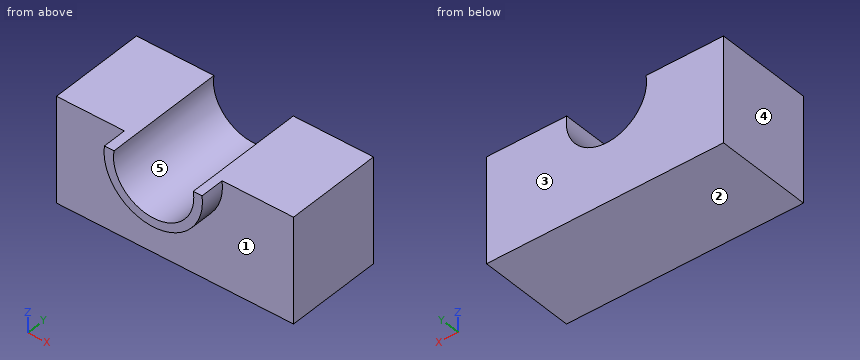
from build123d import *

# Parameters (mm, degrees)
F1_DEPTH = 25.4
F2_R     = 3.02283
F3_DEPTH = 25.4
F5_DEPTH = 6.35


with BuildPart() as f1:
    # F0 (on Front) → F1 (new body)
    with BuildSketch(Plane.XZ):
        with BuildLine():
            Line((-25.424864, 16.508088), (-25.424864, -10.965226))
            Line((-25.424864, -10.965226), (36.510594, -10.965226))
            Line((36.510594, -10.965226), (36.510594, 16.508088))
            Line((36.510594, 16.508088), (19.159023, 16.508088))
            ThreePointArc((19.159023, 16.508088), (5.422366, 0.842331), (-8.314291, 16.508088))
            Line((-8.314291, 16.508088), (-25.424864, 16.508088))
        make_face()
        with BuildLine():
            Line((-5.181369, 16.508088), (-8.314291, 16.508088))
            ThreePointArc((-8.314291, 16.508088), (5.422366, 0.842331), (19.159023, 16.508088))
            Line((19.159023, 16.508088), (15.544111, 16.508088))
            ThreePointArc((15.544111, 16.508088), (5.181371, 4.375351), (-5.181369, 16.508088))
        make_face()
    extrude(amount=F1_DEPTH)

    # F2 (on face) → F3 (join)
    with BuildSketch(Plane.XY.offset(16.508088)):
        with Locations((-15.827941, -12.417181)):
            Circle(F2_R)
    extrude(amount=-F3_DEPTH)

    # F4 (on face) → F5 (join)
    with BuildSketch(Plane.XZ.offset(25.4)):
        with BuildLine():
            ThreePointArc((-7.689733, 16.508088), (5.077277, 2.095446), (17.844288, 16.508088))
            Line((17.844288, 16.508088), (15.544111, 16.508088))
            ThreePointArc((15.544111, 16.508088), (5.181371, 4.375351), (-5.181369, 16.508088))
            Line((-5.181369, 16.508088), (-7.689733, 16.508088))
        make_face()
    extrude(amount=F5_DEPTH)


solid = f1.part
Verification items for the finished model (mm, model axes). Face numbers are marked on the shaded views. A direction names the side the tool comes from. Coordinates: 2 decimals unless noted, no trailing zeros. Order: outer loops, then holes, each group sorted by start corner. A loop starts at its lowest first (then second) coordinate and runs counter-clockwise, first axis right, second up. Notation, with made-up numbers: (-28, 57.5) -> (16, 57.5) arc R28 ccw to (16, 85.5) -> close; hole circle Ø3 at (7, -39). An arc over 180 degrees is marked (long way). Put each result on its own line as item: value. Start each with the question number.
1. Cross-section at C-C, the plane z = -7. Record the boundary of the cut face in (x, y).
2. Material ranges on L1, parallel to Y at x = 25.5, z = 10.75; L2, parallel to X at y = -19, z = 5.75; L3, parallel to X at y = -20.5, z = 13, recorded low to high. Write a range as [from, to].
3. Cross-section at B-B, the plane y = -12.5. Record the boundary of the cut face in (x, z), then the cut area to 3 significant figures.
4. Mould release check, pull along X, two halves, no side actions. Record for the marked faces 3, 4 and 5: released by +X, released by -X, zero draft, split by the parting line, or undercut.
5. Access from +Z, -Z, +X, -X, +Y, -Y to the whole of each face (thin tool, end or side, straight path). Record for the marked faces 1 and 2.
6. Cross-section at A-A, the plane z = 10. Record the boundary of the cut face in (x, y).
7. Cross-section at D-D, the plane x = -11. Record the boundary of the cut face in (y, z).
8. Go/stop test with a flat-tipped pin: pin 1 Ø5 at (x, z) = (13, -8) entering from -Y. Record where the tip stops, or that it passes through.
Computed:
1. outline: (-25.42, -25.4) -> (36.51, -25.4) -> (36.51, 0) -> (-25.42, 0) -> close
2. L1: [-25.4, 0]
2. L2: [-25.42, -0.01], [10.37, 36.51]
2. L3: [-25.42, -5.14], [15.51, 36.51]
3. outline: (-25.42, -10.97) -> (36.51, -10.97) -> (36.51, 16.51) -> (15.54, 16.51) arc R10.49 cw (long way) to (-5.18, 16.51) -> (-25.42, 16.51) -> close
3. area: 1,490 mm2
4. face 3: zero draft
4. face 4: released by -X
4. face 5: undercut
5. face 1: -Z, -Y
5. face 2: -Z, +X, -X, +Y, -Y
6. outline: (-25.42, -25.4) -> (-6.79, -25.4) -> (-6.79, -31.75) -> (-4.11, -31.75) -> (-4.11, 0) -> (-25.42, 0) -> close; (14.48, -31.75) -> (16.94, -31.75) -> (16.94, -25.4) -> (36.51, -25.4) -> (36.51, 0) -> (14.48, 0) -> close
7. outline: (-25.4, -10.97) -> (0, -10.97) -> (0, 16.51) -> (-25.4, 16.51) -> close
8. pin 1: y = -25.4
